Check sheet for the modelled part. Datum: model origin and axes. Units: mm. A direction names the side the tool comes from. Give positions to 0.01 mm unless a question says otherwise; leave off trailing zeros. Write each loop counter-clockwise with the first axis right and the second up, starting at its lowest first coordinate (ties: lowest second). Pieces come first, ordered by that corner, then holes. Notation, with made-up numbers: M 46,46.25 L 76,46.25 A19 cw 76,81.25 Z; hole C 39.5,21.25 d1. An arc over 180 degrees is marked long. Write item = value, one per line. Start each with the question number.
1) Go/stop test with flat-tipped pins: pin 1 (1 mm diameter, centred on x = -25, z = -14, fed in from +Y); pin 2 (6 mm diameter, centred on y = -7.5, z = -5, fed in from -X); pin 3 (4 mm diameter, centred on x = 13.5, z = -16.5, fed in from -Y). Record where each tip stops, or that it passes through.
2) Cross-section at A-A, the plane z = -1. Record the cut outline in (x, y), plus the area to 3 significant figures.
3) Cross-section at B-B, the plane x = 30.5. Record the cut outline in (y, z), plus the area to 3 significant figures.
4) Access from +Z, -Z, +X, -X, +Y, -Y to the whole of each face (thin tool, end or side, straight path). Record for faces 4 (the flat face through (-1, 22.25, -11)), 5 (the flat face through (-1, -22.25, -11)), 6 (the flat face through (0, -24, 0)).
5) Cross-section at C-C, the plane y = 8. Record the cut outline in (x, z).
6) Scan lines: line 1 along Y through (x, z) = (-20, -5.25); line 2 along X through (y, z) = (10, -13.75). Record each from-to range of solid material in increasing order. Write a range as [from, to].
7) Mould release check, pull along X, two halves, no side actions. Record for faces 1 (the flat face through (42.25, 0, -11)), 2 (the flat face through (-42.25, 0, -11)), 3 (the flat face through (-1, 0, 2)): released by +X, released by -X, zero draft, split by the parting line, or undercut.
```python
from build123d import *

# Parameters (mm, degrees)
SKETCH1_W           = 84.5
SKETCH1_H           = 44.5
BOSS_EXTRUDE1_DEPTH = 22.5
SKETCH2_W           = 90.5
SKETCH2_H           = 50.5
BOSS_EXTRUDE2_DEPTH = 2
FILLET1_R           = 1


with BuildPart() as part:
    # Sketch1 → Boss-Extrude1 (new body)
    with BuildSketch(Plane.XY):
        Rectangle(SKETCH1_W, SKETCH1_H)
    extrude(amount=-BOSS_EXTRUDE1_DEPTH)

    # Sketch2 → Boss-Extrude2 (add)
    with BuildSketch(Plane.XY):
        Rectangle(SKETCH2_W, SKETCH2_H)
    extrude(amount=BOSS_EXTRUDE2_DEPTH)

    # Fillet1
    fillet1_edges = [part.edges().sort_by_distance(p)[0] for p in [
        (-42.25, 0, -22.5),
        (-45.25, 0, 2),
        (0, -25.25, 2),
        (45.25, 0, 2),
        (0, 25.25, 2),
        (0, -22.25, -22.5),
        (42.25, 0, -22.5),
        (42.25, -22.25, -11.25),
        (-42.25, -22.25, -11.25),
        (-42.25, 22.25, -11.25),
        (42.25, 22.25, -11.25),
        (0, 22.25, -22.5),
    ]]
    fillet(fillet1_edges, radius=FILLET1_R)


solid = part.part
```
Reply:
q1.pin_1 = 22.25
q1.pin_2 = -42.25
q1.pin_3 = -22.25
q2.outline = M -42.25,-21.25 A1 ccw -41.25,-22.25 L 41.25,-22.25 A1 ccw 42.25,-21.25 L 42.25,21.25 A1 ccw 41.25,22.25 L -41.25,22.25 A1 ccw -42.25,21.25 Z
q2.area = 3,760 mm2
q3.outline = M -25.25,0 L -22.25,0 L -22.25,-21.5 A1 ccw -21.25,-22.5 L 21.25,-22.5 A1 ccw 22.25,-21.5 L 22.25,0 L 25.25,0 L 25.25,1 A1 ccw 24.25,2 L -24.25,2 A1 ccw -25.25,1 Z
q3.area = 1,100 mm2
q4.face_4 = -Z, +X, -X, +Y
q4.face_5 = -Z, +X, -X, -Y
q4.face_6 = -Z
q5.outline = M -45.25,0 L -42.25,0 L -42.25,-21.5 A1 ccw -41.25,-22.5 L 41.25,-22.5 A1 ccw 42.25,-21.5 L 42.25,0 L 45.25,0 L 45.25,1 A1 ccw 44.25,2 L -44.25,2 A1 ccw -45.25,1 Z
q6.line_1 = [-22.25, 22.25]
q6.line_2 = [-42.25, 42.25]
q7.face_1 = released by +X
q7.face_2 = released by -X
q7.face_3 = zero draft
